Geometry check sheet. Reference: drawing and pictorial views, mm from the part's lowest x, y, z. A direction names the side the tool comes from. Round coordinates to 2 decimals unless told otherwise and drop trailing zeros. Order: outer loops, then holes, each group sorted by start corner. A loop starts at its lowest first (then second) coordinate and runs counter-clockwise, first axis right, second up.
Q1. Scan lines: probe 1 along X at (y, z) = (22.5, 4.25); probe 2 along Z at (x, y) = (11, 35); probe 3 along X at (y, z) = (6.5, 9.5). Record each from-to range of solid material in increasing order.
Q2. Set-up check for the marked faces 1 and 2: record each of +Z, -Z, +X, -X, +Y, -Y from which the full face is reachable in a straight line by a thin tool's end or side.
Q3. Cross-section at B-B on y = 14. Record the cut outline in (x, z), then the cut area to 3 significant figures.
Q4. Cross-section at C-C on x = 14.5. Record the cut outline in (y, z).
Q5. Cross-section at A-A on z = 2.5. Record the cut outline in (x, y), then the cut area to 3 significant figures.
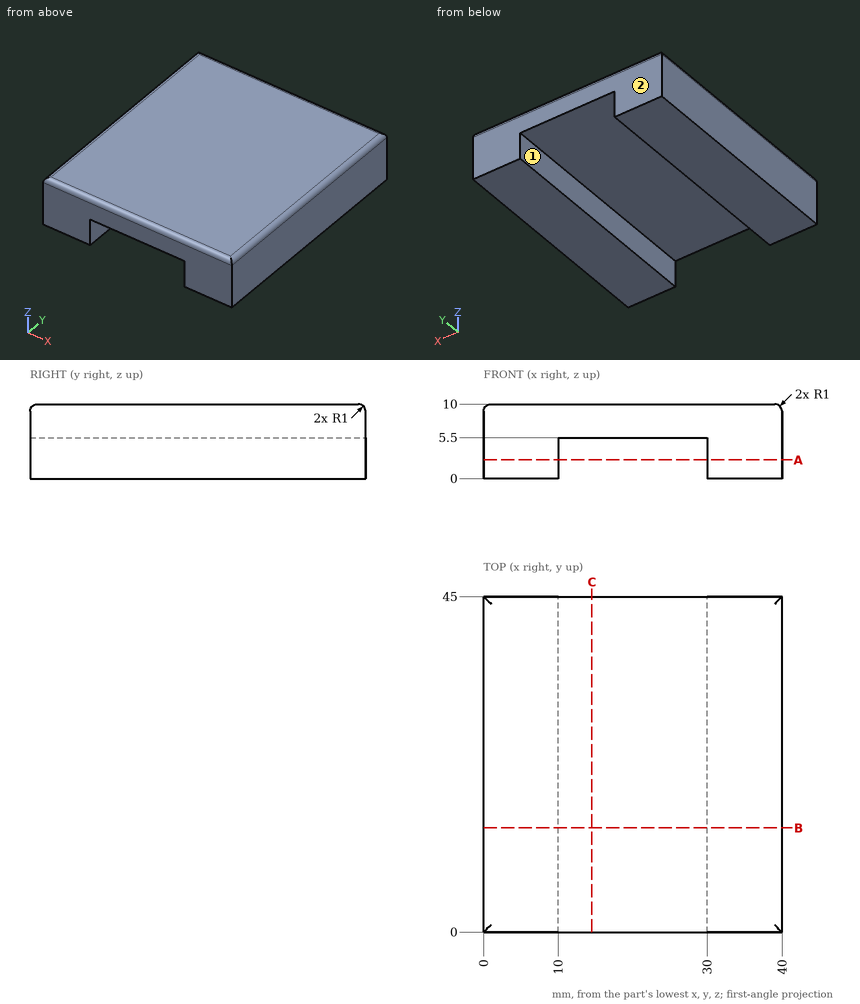
Results found:
1. probe 1: x = 0 to 10, 30 to 40
1. probe 2: z = 5.5 to 10
1. probe 3: x = 0.13 to 39.87
2. face 1: -Z, +Y, -Y
2. face 2: +Z, -Z, +X, -X, +Y
3. outline: (0, 0) - (10, 0) - (10, 5.5) - (30, 5.5) - (30, 0) - (40, 0) - (40, 9) arc R1 ccw to (39, 10) - (1, 10) arc R1 ccw to (0, 9) - close
3. area: 290 mm2
4. outline: (0, 5.5) - (45, 5.5) - (45, 9) arc R1 ccw to (44, 10) - (1, 10) arc R1 ccw to (0, 9) - close
5. outline: (0, 0) - (10, 0) - (10, 45) - (0, 45) - close; (30, 0) - (40, 0) - (40, 45) - (30, 45) - close
5. area: 900 mm2
